```python
from build123d import *

# Parameters (mm, degrees)
F0_R     = 38.1
F1_DEPTH = 25.4


with BuildPart() as f1:
    # F0 (on Front) → F1 (new body)
    with BuildSketch(Plane.XZ):
        with BuildLine():
            ThreePointArc((49.1988245643, 12.6536817364), (50.3981164721, 6.3772922205), (50.8, 0))
            ThreePointArc((50.8, 0), (50.3981164721, -6.3772922205), (49.1988245643, -12.6536817364))
            Line((49.1988245643, -12.6536817364), (49.5602090261, -13.2796179853))
            Line((49.5602090261, -13.2796179853), (72.5611820817, 0))
            Line((72.5611820817, 0), (49.5602090261, 13.2796179853))
            Line((49.5602090261, 13.2796179853), (49.1988245643, 12.6536817364))
        make_face()
        with BuildLine():
            ThreePointArc((48.9342727773, 13.641002447), (49.0690319755, 13.1480074912), (49.1988245643, 12.6536817364))
            Line((49.1988245643, 12.6536817364), (49.5602090261, 13.2796179853))
            Line((49.5602090261, 13.2796179853), (48.9342727773, 13.641002447))
        make_face()
        with BuildLine():
            Line((49.5602090261, -13.2796179853), (49.1988245643, -12.6536817364))
            ThreePointArc((49.1988245643, -12.6536817364), (49.0690319755, -13.1480074912), (48.9342727773, -13.641002447))
            Line((48.9342727773, -13.641002447), (49.5602090261, -13.2796179853))
        make_face()
        with BuildLine():
            ThreePointArc((36.2805910408, 35.5578221173), (43.9940905122, 25.4), (48.9342727773, 13.641002447))
            Line((48.9342727773, 13.641002447), (49.5602090261, 13.2796179853))
            Line((49.5602090261, 13.2796179853), (62.8398270114, 36.2805910408))
            Line((62.8398270114, 36.2805910408), (36.2805910408, 36.2805910408))
            Line((36.2805910408, 36.2805910408), (36.2805910408, 35.5578221173))
        make_face()
        with BuildLine():
            Line((49.5602090261, -13.2796179853), (48.9342727773, -13.641002447))
            ThreePointArc((48.9342727773, -13.641002447), (43.9940905122, -25.4), (36.2805910408, -35.5578221173))
            Line((36.2805910408, -35.5578221173), (36.2805910408, -36.2805910408))
            Line((36.2805910408, -36.2805910408), (62.8398270114, -36.2805910408))
            Line((62.8398270114, -36.2805910408), (49.5602090261, -13.2796179853))
        make_face()
        with BuildLine():
            ThreePointArc((35.5578221173, 36.2805910408), (35.9210244843, 35.9210244843), (36.2805910408, 35.5578221173))
            Line((36.2805910408, 35.5578221173), (36.2805910408, 36.2805910408))
            Line((36.2805910408, 36.2805910408), (35.5578221173, 36.2805910408))
        make_face()
        with BuildLine():
            Line((36.2805910408, -36.2805910408), (36.2805910408, -35.5578221173))
            ThreePointArc((36.2805910408, -35.5578221173), (35.9210244843, -35.9210244843), (35.5578221173, -36.2805910408))
            Line((35.5578221173, -36.2805910408), (36.2805910408, -36.2805910408))
        make_face()
        with BuildLine():
            ThreePointArc((13.641002447, 48.9342727773), (25.4, 43.9940905122), (35.5578221173, 36.2805910408))
            Line((35.5578221173, 36.2805910408), (36.2805910408, 36.2805910408))
            Line((36.2805910408, 36.2805910408), (36.2805910408, 62.8398270114))
            Line((36.2805910408, 62.8398270114), (13.2796179853, 49.5602090261))
            Line((13.2796179853, 49.5602090261), (13.641002447, 48.9342727773))
        make_face()
        with BuildLine():
            Line((36.2805910408, -36.2805910408), (35.5578221173, -36.2805910408))
            ThreePointArc((35.5578221173, -36.2805910408), (25.4, -43.9940905122), (13.641002447, -48.9342727773))
            Line((13.641002447, -48.9342727773), (13.2796179853, -49.5602090261))
            Line((13.2796179853, -49.5602090261), (36.2805910408, -62.8398270114))
            Line((36.2805910408, -62.8398270114), (36.2805910408, -36.2805910408))
        make_face()
        with BuildLine():
            ThreePointArc((12.6536817364, 49.1988245643), (13.1480074912, 49.0690319755), (13.641002447, 48.9342727773))
            Line((13.641002447, 48.9342727773), (13.2796179853, 49.5602090261))
            Line((13.2796179853, 49.5602090261), (12.6536817364, 49.1988245643))
        make_face()
        with BuildLine():
            Line((13.2796179853, -49.5602090261), (13.641002447, -48.9342727773))
            ThreePointArc((13.641002447, -48.9342727773), (13.1480074912, -49.0690319755), (12.6536817364, -49.1988245643))
            Line((12.6536817364, -49.1988245643), (13.2796179853, -49.5602090261))
        make_face()
        with BuildLine():
            ThreePointArc((-12.6536817364, 49.1988245643), (0, 50.8), (12.6536817364, 49.1988245643))
            Line((12.6536817364, 49.1988245643), (13.2796179853, 49.5602090261))
            Line((13.2796179853, 49.5602090261), (0, 72.5611820817))
            Line((0, 72.5611820817), (-13.2796179853, 49.5602090261))
            Line((-13.2796179853, 49.5602090261), (-12.6536817364, 49.1988245643))
        make_face()
        with BuildLine():
            Line((13.2796179853, -49.5602090261), (12.6536817364, -49.1988245643))
            ThreePointArc((12.6536817364, -49.1988245643), (0, -50.8), (-12.6536817364, -49.1988245643))
            Line((-12.6536817364, -49.1988245643), (-13.2796179853, -49.5602090261))
            Line((-13.2796179853, -49.5602090261), (0, -72.5611820817))
            Line((0, -72.5611820817), (13.2796179853, -49.5602090261))
        make_face()
        with BuildLine():
            ThreePointArc((-13.641002447, 48.9342727773), (-13.1480074912, 49.0690319755), (-12.6536817364, 49.1988245643))
            Line((-12.6536817364, 49.1988245643), (-13.2796179853, 49.5602090261))
            Line((-13.2796179853, 49.5602090261), (-13.641002447, 48.9342727773))
        make_face()
        with BuildLine():
            Line((-13.2796179853, -49.5602090261), (-12.6536817364, -49.1988245643))
            ThreePointArc((-12.6536817364, -49.1988245643), (-13.1480074912, -49.0690319755), (-13.641002447, -48.9342727773))
            Line((-13.641002447, -48.9342727773), (-13.2796179853, -49.5602090261))
        make_face()
        with BuildLine():
            ThreePointArc((-35.5578221173, 36.2805910408), (-25.4, 43.9940905122), (-13.641002447, 48.9342727773))
            Line((-13.641002447, 48.9342727773), (-13.2796179853, 49.5602090261))
            Line((-13.2796179853, 49.5602090261), (-36.2805910408, 62.8398270114))
            Line((-36.2805910408, 62.8398270114), (-36.2805910408, 36.2805910408))
            Line((-36.2805910408, 36.2805910408), (-35.5578221173, 36.2805910408))
        make_face()
        with BuildLine():
            Line((-13.2796179853, -49.5602090261), (-13.641002447, -48.9342727773))
            ThreePointArc((-13.641002447, -48.9342727773), (-25.4, -43.9940905122), (-35.5578221173, -36.2805910408))
            Line((-35.5578221173, -36.2805910408), (-36.2805910408, -36.2805910408))
            Line((-36.2805910408, -36.2805910408), (-36.2805910408, -62.8398270114))
            Line((-36.2805910408, -62.8398270114), (-13.2796179853, -49.5602090261))
        make_face()
        with BuildLine():
            ThreePointArc((-36.2805910408, 35.5578221173), (-35.9210244843, 35.9210244843), (-35.5578221173, 36.2805910408))
            Line((-35.5578221173, 36.2805910408), (-36.2805910408, 36.2805910408))
            Line((-36.2805910408, 36.2805910408), (-36.2805910408, 35.5578221173))
        make_face()
        with BuildLine():
            Line((-36.2805910408, -36.2805910408), (-35.5578221173, -36.2805910408))
            ThreePointArc((-35.5578221173, -36.2805910408), (-35.9210244843, -35.9210244843), (-36.2805910408, -35.5578221173))
            Line((-36.2805910408, -35.5578221173), (-36.2805910408, -36.2805910408))
        make_face()
        with BuildLine():
            ThreePointArc((-48.9342727773, 13.641002447), (-43.9940905122, 25.4), (-36.2805910408, 35.5578221173))
            Line((-36.2805910408, 35.5578221173), (-36.2805910408, 36.2805910408))
            Line((-36.2805910408, 36.2805910408), (-62.8398270114, 36.2805910408))
            Line((-62.8398270114, 36.2805910408), (-49.5602090261, 13.2796179853))
            Line((-49.5602090261, 13.2796179853), (-48.9342727773, 13.641002447))
        make_face()
        with BuildLine():
            Line((-36.2805910408, -36.2805910408), (-36.2805910408, -35.5578221173))
            ThreePointArc((-36.2805910408, -35.5578221173), (-43.9940905122, -25.4), (-48.9342727773, -13.641002447))
            Line((-48.9342727773, -13.641002447), (-49.5602090261, -13.2796179853))
            Line((-49.5602090261, -13.2796179853), (-62.8398270114, -36.2805910408))
            Line((-62.8398270114, -36.2805910408), (-36.2805910408, -36.2805910408))
        make_face()
        with BuildLine():
            ThreePointArc((-49.1988245643, 12.6536817364), (-49.0690319755, 13.1480074912), (-48.9342727773, 13.641002447))
            Line((-48.9342727773, 13.641002447), (-49.5602090261, 13.2796179853))
            Line((-49.5602090261, 13.2796179853), (-49.1988245643, 12.6536817364))
        make_face()
        with BuildLine():
            Line((-49.5602090261, -13.2796179853), (-48.9342727773, -13.641002447))
            ThreePointArc((-48.9342727773, -13.641002447), (-49.0690319755, -13.1480074912), (-49.1988245643, -12.6536817364))
            Line((-49.1988245643, -12.6536817364), (-49.5602090261, -13.2796179853))
        make_face()
        with BuildLine():
            ThreePointArc((-49.1988245643, -12.6536817364), (-50.8, 0), (-49.1988245643, 12.6536817364))
            Line((-49.1988245643, 12.6536817364), (-49.5602090261, 13.2796179853))
            Line((-49.5602090261, 13.2796179853), (-72.5611820817, 0))
            Line((-72.5611820817, 0), (-49.5602090261, -13.2796179853))
            Line((-49.5602090261, -13.2796179853), (-49.1988245643, -12.6536817364))
        make_face()
        with BuildLine():
            ThreePointArc((49.1988245643, -12.6536817364), (50.3981164721, -6.3772922205), (50.8, 0))
            ThreePointArc((50.8, 0), (50.3981164721, 6.3772922205), (49.1988245643, 12.6536817364))
            ThreePointArc((49.1988245643, 12.6536817364), (49.0690319755, 13.1480074912), (48.9342727773, 13.641002447))
            ThreePointArc((48.9342727773, 13.641002447), (43.9940905122, 25.4), (36.2805910408, 35.5578221173))
            ThreePointArc((36.2805910408, 35.5578221173), (35.9210244843, 35.9210244843), (35.5578221173, 36.2805910408))
            ThreePointArc((35.5578221173, 36.2805910408), (25.4, 43.9940905122), (13.641002447, 48.9342727773))
            ThreePointArc((13.641002447, 48.9342727773), (13.1480074912, 49.0690319755), (12.6536817364, 49.1988245643))
            ThreePointArc((12.6536817364, 49.1988245643), (0, 50.8), (-12.6536817364, 49.1988245643))
            ThreePointArc((-12.6536817364, 49.1988245643), (-13.1480074912, 49.0690319755), (-13.641002447, 48.9342727773))
            ThreePointArc((-13.641002447, 48.9342727773), (-25.4, 43.9940905122), (-35.5578221173, 36.2805910408))
            ThreePointArc((-35.5578221173, 36.2805910408), (-35.9210244843, 35.9210244843), (-36.2805910408, 35.5578221173))
            ThreePointArc((-36.2805910408, 35.5578221173), (-43.9940905122, 25.4), (-48.9342727773, 13.641002447))
            ThreePointArc((-48.9342727773, 13.641002447), (-49.0690319755, 13.1480074912), (-49.1988245643, 12.6536817364))
            ThreePointArc((-49.1988245643, 12.6536817364), (-50.8, 0), (-49.1988245643, -12.6536817364))
            ThreePointArc((-49.1988245643, -12.6536817364), (-49.0690319755, -13.1480074912), (-48.9342727773, -13.641002447))
            ThreePointArc((-48.9342727773, -13.641002447), (-43.9940905122, -25.4), (-36.2805910408, -35.5578221173))
            ThreePointArc((-36.2805910408, -35.5578221173), (-35.9210244843, -35.9210244843), (-35.5578221173, -36.2805910408))
            ThreePointArc((-35.5578221173, -36.2805910408), (-25.4, -43.9940905122), (-13.641002447, -48.9342727773))
            ThreePointArc((-13.641002447, -48.9342727773), (-13.1480074912, -49.0690319755), (-12.6536817364, -49.1988245643))
            ThreePointArc((-12.6536817364, -49.1988245643), (0, -50.8), (12.6536817364, -49.1988245643))
            ThreePointArc((12.6536817364, -49.1988245643), (13.1480074912, -49.0690319755), (13.641002447, -48.9342727773))
            ThreePointArc((13.641002447, -48.9342727773), (25.4, -43.9940905122), (35.5578221173, -36.2805910408))
            ThreePointArc((35.5578221173, -36.2805910408), (35.9210244843, -35.9210244843), (36.2805910408, -35.5578221173))
            ThreePointArc((36.2805910408, -35.5578221173), (43.9940905122, -25.4), (48.9342727773, -13.641002447))
            ThreePointArc((48.9342727773, -13.641002447), (49.0690319755, -13.1480074912), (49.1988245643, -12.6536817364))
        make_face()
        Circle(F0_R, mode=Mode.SUBTRACT)
        Circle(F0_R)
    extrude(amount=F1_DEPTH)


solid = f1.part
```
Source: CAD feature listing. Evaluate the final solid. Frame: model axes, mm. A direction names the side the tool comes from. Give positions to 0.01 mm unless a question says otherwise; leave off trailing zeros. Order: outer loops, then holes, each group sorted by start corner. A loop starts at its lowest first (then second) coordinate and runs counter-clockwise, first axis right, second up. Notation, with made-up numbers: (29, -39) -> (57, -39) arc R26 cw to (57, -14) -> close; hole circle Ø6 at (2.25, 41.5). An arc over 180 degrees is marked (long way). Use a Markdown table: item, result.
Q1. First-contact query: P1, Ø4, axis at x = -41.5, y = -21, coming from the -Z side; P2, Ø7.5, axis at x = 54, y = -17.5, coming from the +Z side; P3, Ø10, axis at y = -22.5, z = 42.5, coming from the +X side. Flat tips, straight axial feed; report the tip coordinate or a pass-through.
A:
| item | result |
|---|---|
| P1 | z = -36.28 |
| P2 | z = 36.28 |
| P3 | x = 36.28 |
Q2. Section B-B (y = -11.25). Return the cut outline in (x, z).
A:
| item | result |
|---|---|
| outline | (-72.56, 0) -> (-49.56, -13.28) -> (-62.84, -36.28) -> (-36.28, -36.28) -> (-36.28, -62.84) -> (-13.28, -49.56) -> (0, -72.56) -> (13.28, -49.56) -> (36.28, -62.84) -> (36.28, -36.28) -> (62.84, -36.28) -> (49.56, -13.28) -> (72.56, 0) -> (49.56, 13.28) -> (62.84, 36.28) -> (36.28, 36.28) -> (36.28, 62.84) -> (13.28, 49.56) -> (0, 72.56) -> (-13.28, 49.56) -> (-36.28, 62.84) -> (-36.28, 36.28) -> (-62.84, 36.28) -> (-49.56, 13.28) -> close |
Q3. Section C-C (z = -40). Return the cut outline in (x, y), and give its area (3 significant figures).
A:
| item | result |
|---|---|
| outline | (-36.28, -25.4) -> (36.28, -25.4) -> (36.28, 0) -> (-36.28, 0) -> close |
| area | 1,840 mm^2 |
Q4. Pull-direction query (X, two-part tool) for faces 6 (the face through (-6.55, -12.52, 61.22)), 7 (the face through (-61.22, -12.52, -6.55)), 8 (the face through (24.619, -12.522, -56.107)), 9 (the face through (-1, 0, 1)); classes: +X half, -X half, draft (parallel to the pull), parting line (faces both ways), or undercut.
A:
| item | result |
|---|---|
| face 6 | undercut |
| face 7 | -X half |
| face 8 | undercut |
| face 9 | draft |
Q5. Section D-D (x = 4). Return the cut outline in (y, z).
A:
| item | result |
|---|---|
| outline | (-25.4, -65.63) -> (0, -65.63) -> (0, 65.63) -> (-25.4, 65.63) -> close |
Q6. Access query for faces 1 (the face through (49, -13, -36.281)), 2 (the face through (61.22, -12.52, 6.55)), 3 (the face through (-24.941, -12.522, -56.293)), 4 (the face through (-56.107, -12.522, -24.619)), 5 (the face through (-50, -13, -36.281)). Directions: +Z, -Z, +X, -X, +Y, -Y. A direction counts if a zero-diameter tool reaches every point of the face in a straight line with its end or side. Return the directions, or none.
A:
| item | result |
|---|---|
| face 1 | -Z, +X, +Y, -Y |
| face 2 | +X, +Y, -Y |
| face 3 | -Z, +Y, -Y |
| face 4 | -X, +Y, -Y |
| face 5 | -Z, -X, +Y, -Y |
Q7. Section A-A (z = 56.5). Return the cut outline in (x, y), and give its area (3 significant figures).
A:
| item | result |
|---|---|
| outline | (-36.28, -25.4) -> (-25.3, -25.4) -> (-25.3, 0) -> (-36.28, 0) -> close; (-9.27, -25.4) -> (9.27, -25.4) -> (9.27, 0) -> (-9.27, 0) -> close; (25.3, -25.4) -> (36.28, -25.4) -> (36.28, 0) -> (25.3, 0) -> close |
| area | 1,030 mm^2 |
Q8. Material intervals for line 1 (X direction, y = -15, z = -56); line 2 (Z direction, x = 54.5, y = -20); line 3 (Z direction, x = 56.5, y = -3.75), sorted ascending. Write a range as [from, to].
A:
| item | result |
|---|---|
| line 1 | [-36.28, -24.43], [-9.56, 9.56], [24.43, 36.28] |
| line 2 | [-36.28, -21.84], [-10.43, 10.43], [21.84, 36.28] |
| line 3 | [-36.28, -25.3], [-9.27, 9.27], [25.3, 36.28] |
